Geometry: see drawing. Coordinates: mm, zero at the bounding-box minimum. A direction names the side the tool comes from. Coordinates: 2 decimals unless noted, no trailing zeros. Write each loop counter-clockwise with the first axis right and the second up, starting at its lowest first coordinate (ties: lowest second). Pieces come first, ordered by that corner, then holes. Notation, with made-up numbers: M 0,4.25 L 57,4.25 A18 cw 57,18.25 Z; hole C 33,0.5 d4. An arc over 180 degrees is marked long. One line per item, written item: value. Start each with the question number.
Item 1: Cut plane D-D, the plane y = 10.5. Output: boundary loops of the cut face in (x, z), then the cut area to 3 significant figures.
Item 2: Cut plane A-A, the plane z = 4. Output: boundary loops of the cut face in (x, y), then the cut area to 3 significant figures.
Item 3: Set-up query: the marked faces 1 and 2. Return all of +Z, -Z, +X, -X, +Y, -Y with unobstructed straight access to the full face (end or side cutting, diameter ignored); none if empty.
Item 4: Pin query (flat end, axial travel): P1, Ø1.5, axis at x = 5.5, z = 6, coming from the -Y side; P2, Ø1.5, axis at y = 8.5, z = 3, coming from the +X side; P3, Ø1.5, axis at x = 3, y = 15, coming from the -Z side. Return the tip coordinate at first contact, or that it passes through.
Item 5: Cut plane C-C, the plane y = 2. Output: boundary loops of the cut face in (x, z), then the cut area to 3 significant figures.
Item 6: Ray query, L1, parallel to Y at x = 1.25, z = 4.25; L2, parallel to Z at x = 5, y = 11.25. Return the intervals inside material, ascending. Write a range as from..to.
Item 7: Cut plane B-B, the plane x = 4. Output: boundary loops of the cut face in (y, z), then the cut area to 3 significant figures.
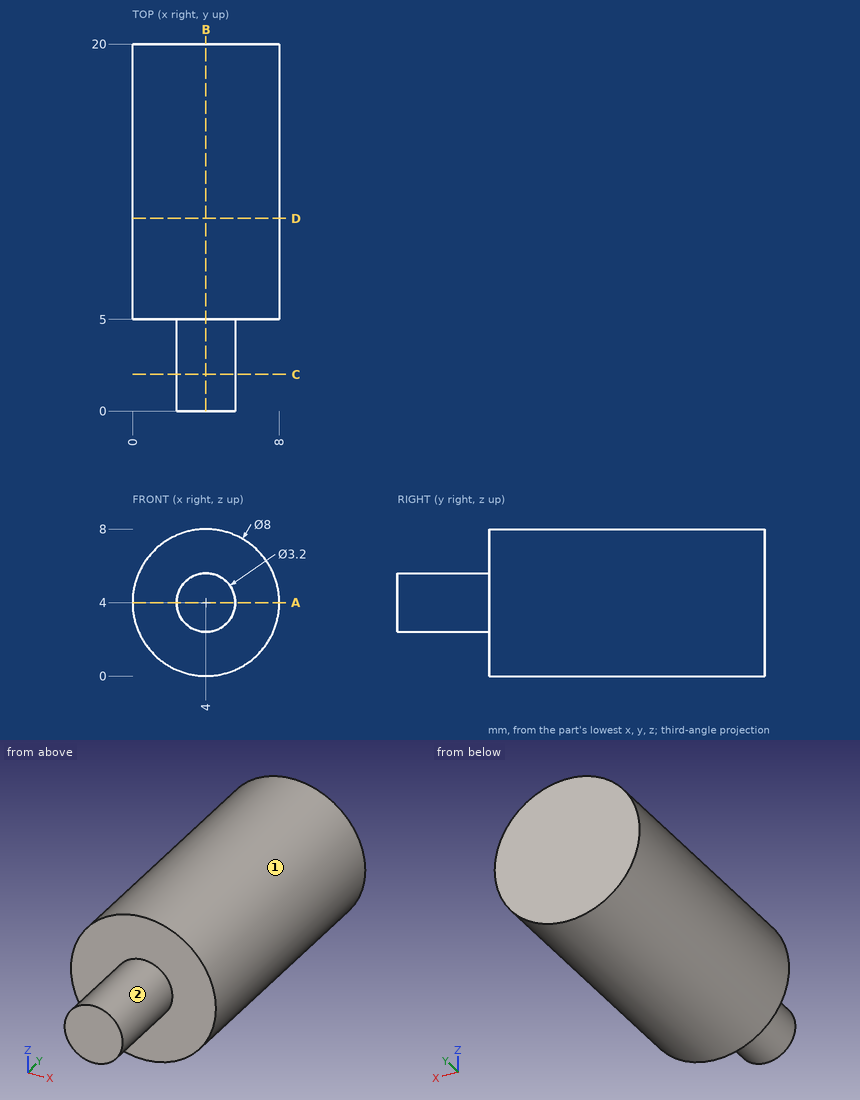
From the geometry:
1. outline: C 4,4 d8
1. area: 50.3 mm²
2. outline: M 0,5 L 2.4,5 L 2.4,0 L 5.6,0 L 5.6,5 L 8,5 L 8,20 L 0,20 Z
2. area: 136 mm²
3. face 1: +Y, -Y
3. face 2: -Y
4. P1: stops at y = 5
4. P2: stops at x = 7.99
4. P3: stops at z = 0.01
5. outline: C 4,4 d3.2
5. area: 8.04 mm²
6. L1: y = 5..20
6. L2: z = 0.13..7.87
7. outline: M 0,2.4 L 5,2.4 L 5,0 L 20,0 L 20,8 L 5,8 L 5,5.6 L 0,5.6 Z
7. area: 136 mm²
